Job drawing, mm, ordinate dimensions from the low corner. One solid piece. A direction names the side the tool comes from. Coordinates: 2 decimals unless noted, no trailing zeros. Loops run counter-clockwise (first coordinate to the right, second up) from the corner with the lowest first, then second, coordinate; pieces in that order, holes last. Notation, with made-up numbers: (-31, 68.5) - (14, 68.5) arc R14 ccw to (14, 85.5) - close; hole circle Ø8 at (67, 21.25). An arc over 180 degrees is marked (long way). Use a Markdown table: item, result. Add a question column.
1. Band-saw the part on D-D, the plane y = 4. Give the cut face in (x, z).
2. Band-saw the part on B-B, the plane z = 34. Give the cut face in (x, y), plus the area to 3 significant figures.
3. Wall check: probe 1 along Y at (x, z) = (18, 30); probe 2 along Y at (x, z) = (5, 3); probe 3 along X at (y, z) = (13, 22). Give the ranges that are in metal, low to high. Write a range as [from, to].
4. Band-saw the part on C-C, the plane z = 3. Give the cut face in (x, y).
5. 3-axis set-ups, long thin cutter, end or side, ignore diameter. For the marked faces 1, 2 and 3: which of +Z, -Z, +X, -X, +Y, -Y reach the whole face in a straight line?
6. Band-saw the part on A-A, the plane y = 20. Give the cut face in (x, z).
7. Drop flat-ended pins along their axis: pin 1 (2.5 mm diameter, centred on x = 5, y = 5, fed in from +Z); pin 2 (4.5 mm diameter, centred on x = 3.5, y = 27, fed in from +Z); pin 3 (1 mm diameter, centred on x = 18.5, y = 15, fed in from +Z); pin 4 (10.5 mm diameter, centred on y = 19.5, z = 25.5, fed in from +X). Give the stop position or say it passes through.
8. Pull direction Y, two halves, no side cores. Call the marked faces 4, 5 and 6: pulls with the +Y half, pulls with the -Y half, needs draft (parallel to the pull), parting line crosses it, or undercut.
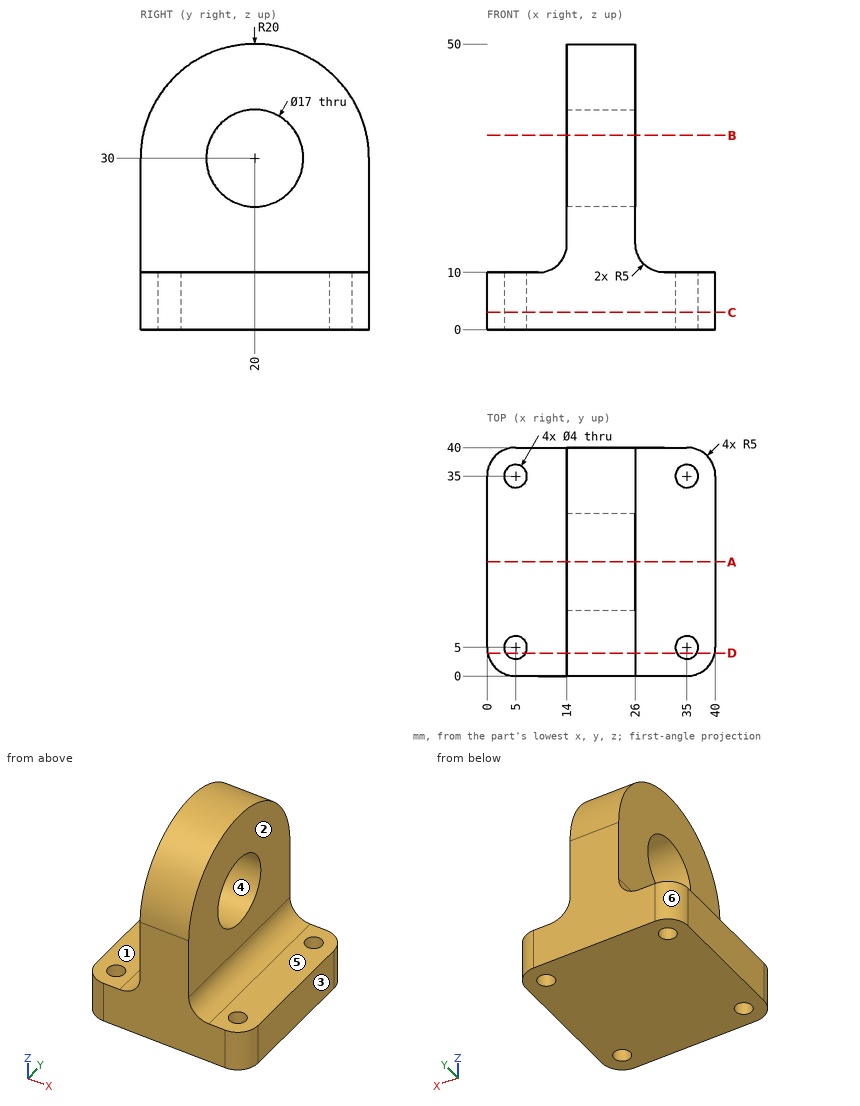
Geometry check:
| question | item | result |
|---|---|---|
| 1 | outline | (0.1, 0) - (3.27, 0) - (3.27, 10) - (0.1, 10) - close; (6.73, 0) - (33.27, 0) - (33.27, 10) - (31, 10) arc R5 cw to (26, 15) - (26, 42) - (14, 42) - (14, 15) arc R5 cw to (9, 10) - (6.73, 10) - close; (36.73, 0) - (39.9, 0) - (39.9, 10) - (36.73, 10) - close |
| 2 | outline | (14, 0.4) - (26, 0.4) - (26, 12.5) - (14, 12.5) - close; (14, 27.5) - (26, 27.5) - (26, 39.6) - (14, 39.6) - close |
| 2 | area | 290 mm^2 |
| 3 | probe 1 | y = [0, 11.5], [28.5, 40] |
| 3 | probe 2 | y = [0, 3], [7, 33], [37, 40] |
| 3 | probe 3 | x = [14, 26] |
| 4 | outline | (0, 5) arc R5 ccw to (5, 0) - (35, 0) arc R5 ccw to (40, 5) - (40, 35) arc R5 ccw to (35, 40) - (5, 40) arc R5 ccw to (0, 35) - close; hole circle Ø4 at (5, 5); hole circle Ø4 at (5, 35); hole circle Ø4 at (35, 5); hole circle Ø4 at (35, 35) |
| 5 | face 1 | +Z, -X, +Y, -Y |
| 5 | face 2 | +Z, +X, +Y, -Y |
| 5 | face 3 | +Z, -Z, +X, +Y, -Y |
| 6 | outline | (0, 0) - (40, 0) - (40, 10) - (31, 10) arc R5 cw to (26, 15) - (26, 21.5) - (14, 21.5) - (14, 15) arc R5 cw to (9, 10) - (0, 10) - close; (14, 38.5) - (26, 38.5) - (26, 50) - (14, 50) - close |
| 7 | pin 1 | passes through |
| 7 | pin 2 | stops at z = 10 |
| 7 | pin 3 | stops at z = 49.49 |
| 7 | pin 4 | stops at x = 26 |
| 8 | face 4 | undercut |
| 8 | face 5 | needs draft |
| 8 | face 6 | pulls with the +Y half |
